from build123d import *

# Parameters (mm, degrees)
F0_R     = 76.6222869854
F0_R_2   = 36.4455054166
F1_DEPTH = 25.4
F2_T     = -2.54
F3_R     = 5.08


with BuildPart() as f1:
    # F0 (on Top) → F1 (new body)
    with BuildSketch(Plane.XY):
        Circle(F0_R)
        Circle(F0_R_2, mode=Mode.SUBTRACT)
    extrude(amount=F1_DEPTH)

    # F2
    f2_openings = [f1.faces().sort_by_distance(p)[0] for p in [
        (-74.455081, 0, 25.4),
    ]]
    offset(amount=F2_T, openings=f2_openings)

    # F3
    f3_edges = [f1.edges().sort_by_distance(p)[0] for p in [
        (-74.082287, 0, 2.54),
        (-38.985505, 0, 2.54),
    ]]
    fillet(f3_edges, radius=F3_R)


solid = f1.part
Check sheet for the modelled part. Datum: model origin and axes. Units: mm. A direction names the side the tool comes from. Round coordinates to 2 decimals unless told otherwise and drop trailing zeros. Loops run counter-clockwise (first coordinate to the right, second up) from the corner with the lowest first, then second, coordinate; pieces in that order, holes last. Notation, with made-up numbers: M 54.25,24 L 110.25,24 A8 cw 110.25,35 Z; hole C 17,-19.5 d10. An arc over 180 degrees is marked long. One line per question, with ' | ' between items. Start each with the question number.
Item 1: Set-up check for faces 1 (the face through (26, -26, 25.4)), 2 (the face through (-58.79, -45.08, 16.39)): record each of +Z, -Z, +X, -X, +Y, -Y from which the full face is reachable in a straight line by a thin tool's end or side.
Item 2: Scan lines: probe 1 along Y at (x, z) = (0, 9.5); probe 2 along X at (y, z) = (12, 13.5); probe 3 along Y at (x, z) = (-11, 20.25). Record each from-to range of solid material in increasing order.
Item 3: Section check A-A (z = 14). Record the boundary of the cut face in (x, y), and give its area (3 significant figures).
Item 4: Section check B-B (x = 0). Record the boundary of the cut face in (y, z).
Item 5: Gauge pin test, flat ends, axial feed: pin 1 Ø2 at (x, z) = (-10, 9) entering from -Y; pin 2 Ø10 at (x, y) = (12, 50.5) entering from -Z; pin 3 Ø2 at (x, y) = (-30.5, -52.5) entering from +Z; pin 4 Ø1.5 at (x, z) = (-9, 19) entering from +Y. Record the tip position at first contact, or that the pin passes through.
Item 6: Release check for a two-part mould opening along X. For faces 3 (the face through (-4.744, 36.135, 12.522)), 4 (the face through (16, -33, 0)), 5 (the face through (70.8, -29.3, 12.5)) record: released by +X, released by -X, zero draft, split by the parting line, or undercut.
Worked out:
1) face 1: +Z, +X, -X, +Y, -Y | face 2: +Z
2) probe 1: -76.62 to -74.08, -38.99 to -36.45, 36.45 to 38.99, 74.08 to 76.62 | probe 2: -75.68 to -73.1, -37.09 to -34.41, 34.41 to 37.09, 73.1 to 75.68 | probe 3: -75.83 to -73.26, -37.4 to -34.75, 34.75 to 37.4, 73.26 to 75.83
3) outline: C 0,0 d153.24; C 0,0 d77.97; hole C 0,0 d148.16; hole C 0,0 d72.89 | area: 1,800 mm^2
4) outline: M -76.62,0 L -36.45,0 L -36.45,25.4 L -38.99,25.4 L -38.99,7.62 A5.08 cw -44.07,2.54 L -69,2.54 A5.08 cw -74.08,7.62 L -74.08,25.4 L -76.62,25.4 Z; M 36.45,0 L 76.62,0 L 76.62,25.4 L 74.08,25.4 L 74.08,7.62 A5.08 cw 69,2.54 L 44.07,2.54 A5.08 cw 38.99,7.62 L 38.99,25.4 L 36.45,25.4 Z
5) pin 1: y = -76.09 | pin 2: z = 0 | pin 3: z = 2.54 | pin 4: y = 76.18
6) face 3: undercut | face 4: zero draft | face 5: split by the parting line
